from build123d import *

# Parameters (mm, degrees)
EXTRUDE_1_DEPTH        = 8
HOLE_WIZARD_M4_1_D     = 4.3
HOLE_WIZARD_M4_1_DEPTH = 5
HOLE_WIZARD_M4_1_2_D   = 3.3
HOLE_WIZARD_M3_1_D     = 2.5
HOLE_WIZARD_M3_1_DEPTH = 8.5
HOLE_WIZARD_M3_1_TIP   = 0.751075774


with BuildPart() as part:
    # 草图1 → 凸台-拉伸1 (new, symmetric)
    with BuildSketch(Plane(origin=(0, 0, 0), x_dir=(0, 0, -1), z_dir=(1, 0, 0))):
        Polygon((-11, 32), (-11, 3), (11, 3), (11, 32), (16, 32), (16, 0), (-16, 0), (-16, 32), align=None)
    extrude(amount=EXTRUDE_1_DEPTH, both=True)

    # Hole Wizard M4 _1
    with Locations(Plane.XY.offset(16)):
        with Locations((0, 29)):
            Hole(HOLE_WIZARD_M4_1_D / 2, depth=HOLE_WIZARD_M4_1_DEPTH)

    # Hole Wizard M4 _1 2 (through all)
    with Locations(Plane(origin=(0, 0, -16), x_dir=(-1, 0, 0), z_dir=(0, 0, -1))):
        with Locations((0, 29)):
            Hole(HOLE_WIZARD_M4_1_2_D / 2)

    # M3 螺纹孔1
    with Locations(Plane(origin=(0, 0, 0), x_dir=(-1, 0, 0), z_dir=(0, -1, 0))):
        with Locations((0, 13.5), (0, -13.5)):
            Hole(HOLE_WIZARD_M3_1_D / 2, depth=HOLE_WIZARD_M3_1_DEPTH)
            with Locations((0, 0, -(HOLE_WIZARD_M3_1_DEPTH + HOLE_WIZARD_M3_1_TIP / 2))):  # 118° drill point
                Cone(0, HOLE_WIZARD_M3_1_D / 2, HOLE_WIZARD_M3_1_TIP, mode=Mode.SUBTRACT)


solid = part.part
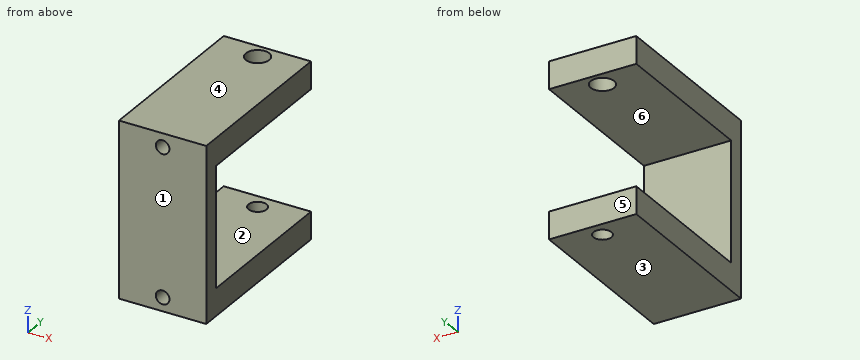
Can you work these out from the model? Positions are in its coordinate system, mm. Face numbers are marked on the shaded views. A direction names the side the tool comes from. Coordinates: 2 decimals unless noted, no trailing zeros. Order: outer loops, then holes, each group sorted by start corner. A loop starts at its lowest first (then second) coordinate and runs counter-clockwise, first axis right, second up. Notation, with made-up numbers: (31, 38.5) - (77, 38.5) arc R16 ccw to (77, 64.5) - close; hole circle Ø9 at (-36, -10.75). An arc over 180 degrees is marked (long way). Answer as a JSON object with one key per item and string values. Group by question number.
Q1. Imagine slicing it at B-B (y = 29). Please give me the cut outline in (x, z), and give its area (3 significant figures).
Q2. We'd pull the mould along Z, two halves only. Please class the marked faces 1, 2, 3 and 4: +Z half, -Z half, draft (parallel to the pull), parting line (faces both ways), or undercut.
Q3. On a 3-axis mill with a long thin cutter (end or side, diameter ignored), from which of +Z, -Z, +X, -X, +Y, -Y can I reach the whole of each face in a straight line? I mean the marked faces 5 and 6. Say none if no direction works.
Q4. I need wall thicknesses on line 1 (Z direction, x = 0, y = 5.75); line 2 (Z direction, x = 4, y = 26); line 3 (X direction, y = 2.25, z = 13.5). Which ranges of each line are inside material? Lowest first, please. Write a range as from..to.
Q5. Will these pins go through, and if not, where does the flat tip stop? P1, Ø4, axis at x = 5, z = 2, coming from the +Y side; P2, Ø2, axis at x = 0, z = 13.5, coming from the -Y side.
Q6. Imagine slicing it at A-A (y = 8). Please give me the cut outline in (x, z).
Q7. Imagine slicing it at C-C (y = 14). Please give me the cut outline in (x, z), and give its area (3 significant figures).
Q8. Imagine slicing it at D-D (x = 5.75). Please give me the cut outline in (y, z), and give its area (3 significant figures).
Determined:
{
 "1": {"outline": "(-8, -16) - (-1.65, -16) - (-1.65, -11) - (-8, -11) - close; (-8, 11) - (-2.15, 11) - (-2.15, 16) - (-8, 16) - close; (1.65, -16) - (8, -16) - (8, -11) - (1.65, -11) - close; (2.15, 11) - (8, 11) - (8, 16) - (2.15, 16) - close", "area": "122 mm2"},
 "2": {"face 1": "draft", "face 2": "undercut", "face 3": "-Z half", "face 4": "+Z half"},
 "3": {"face 5": "+Z, -Z, +X, -X, +Y", "face 6": "+X, -X, +Y"},
 "4": {"line 1": "z = -16..-14.75, -12.25..-11, 11..12.25, 14.75..16", "line 2": "z = -16..-11, 11..16", "line 3": "x = -8..-1.25, 1.25..8"},
 "5": {"P1": "stops at y = 3", "P2": "stops at y = 8.65"},
 "6": {"outline": "(-8, -16) - (8, -16) - (8, -11) - (-8, -11) - close; (-8, 11) - (8, 11) - (8, 16) - (-8, 16) - close; hole circle Ø2.5 at (0, -13.5); hole circle Ø2.5 at (0, 13.5)"},
 "7": {"outline": "(-8, -16) - (8, -16) - (8, -11) - (-8, -11) - close; (-8, 11) - (8, 11) - (8, 16) - (-8, 16) - close", "area": "160 mm2"},
 "8": {"outline": "(0, -16) - (32, -16) - (32, -11) - (3, -11) - (3, 11) - (32, 11) - (32, 16) - (0, 16) - close", "area": "386 mm2"}
}
